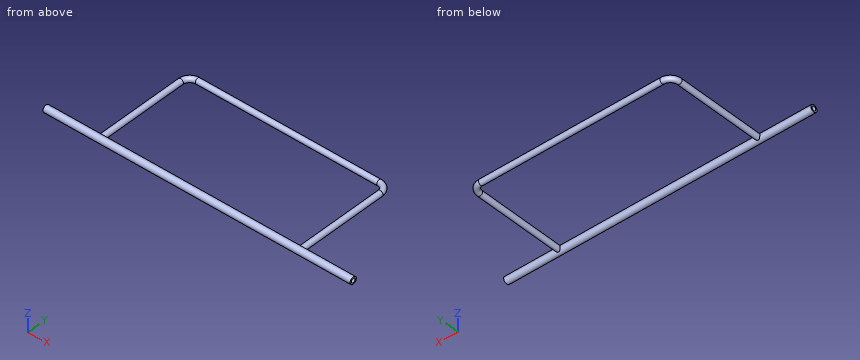
```python
from build123d import *

# Parameters (mm, degrees)
SKETCH1_R           = 5
BOSS_EXTRUDE1_DEPTH = 220
SWEEP1_PROFILE_R    = 4
SKETCH9_R           = 3
CUT_EXTRUDE1_DEPTH  = 220


with BuildPart() as part:
    # Sketch1 → Boss-Extrude1 (new body)
    with BuildSketch(Plane(origin=(0, 0, 0), x_dir=(0, 0, -1), z_dir=(1, 0, 0))):
        Circle(SKETCH1_R)
    boss_extrude1 = extrude(amount=-BOSS_EXTRUDE1_DEPTH)

    # Sweep1: sweep along a path in Sketch2
    with BuildLine(Plane.XY) as sweep1_path:
        Line((-143, 0), (-143, 130))
        ThreePointArc((-143, 130), (-139.192388155, 139.192388155), (-130, 143))
        Line((-130, 143), (0, 143))
    # Sweep1 profile (on start of the path) → Sweep1 (sweep)
    with BuildSketch(Plane(origin=(-143, 0, 0), x_dir=(0, 0, 1), z_dir=(0, 1, 0))):
        Circle(SWEEP1_PROFILE_R)
    sweep1 = sweep(path=sweep1_path.line)

    # Sketch9 → Cut-Extrude1 (cut)
    with BuildSketch(Plane(origin=(0, 0, 0), x_dir=(0, 0, -1), z_dir=(1, 0, 0))):
        Circle(SKETCH9_R)
    cut_extrude1 = extrude(amount=-CUT_EXTRUDE1_DEPTH, mode=Mode.SUBTRACT)

    # Mirror1: Boss-Extrude1, Sweep1, Cut-Extrude1 across plane
    add(boss_extrude1.mirror(Plane(origin=(0, 0, 0), x_dir=(0, 0, 1), z_dir=(1, 0, 0))))
    add(sweep1.mirror(Plane(origin=(0, 0, 0), x_dir=(0, 0, 1), z_dir=(1, 0, 0))))
    add(cut_extrude1.mirror(Plane(origin=(0, 0, 0), x_dir=(0, 0, 1), z_dir=(1, 0, 0))), mode=Mode.SUBTRACT)


solid = part.part
```
Input: part model. Units: mm. Frame: model coordinates. Give positions to 0.01 mm unless a question says otherwise; leave off trailing zeros. Write each loop counter-clockwise with the first axis right and the second up, starting at its lowest first coordinate (ties: lowest second). Pieces come first, ordered by that corner, then holes. Notation, with made-up numbers: (63, -8) - (102, -8) arc R21 cw to (102, 14) - close; hole circle Ø6 at (85.5, 29). An arc over 180 degrees is marked (long way). Write item = value, one per line. Start each with the question number.
1) Cut plane D-D (x = -193). Return loops of the section in (y, z), and give its area (3 significant figures).
2) Cut plane A-A (z = 0). Return loops of the section in (x, y).
3) Cut plane B-B (x = -119.5). Return loops of the section in (y, z).
4) Material intervals for L1, parallel to Y at x = 114, z = 0.5; L2, parallel to Y at x = -137, z = 0; L3, parallel to X at y = 21, z = 0, sorted ascending. Write a range as [from, to].
5) Pin query (flat end, axial travel): pin 1 (1 mm diameter, centred on x = -11.5, z = -2, fed in from -Y); pin 2 (1.5 mm diameter, centred on y = 96.5, z = -3, fed in from -X). Return the tip coordinate at first contact, or that it passes through.
6) Cut plane C-C (y = 74). Return loops of the section in (x, z), and give its area (3 significant figures).
Answers follow:
q1.outline = circle Ø10 at (0, 0); hole circle Ø6 at (0, 0)
q1.area = 50.3 mm^2
q2.outline = (-220, -5) - (220, -5) - (220, -3) - (-220, -3) - close; (-220, 3) - (220, 3) - (220, 5) - (147, 5) - (147, 130) arc R17 ccw to (130, 147) - (-130, 147) arc R17 ccw to (-147, 130) - (-147, 5) - (-220, 5) - close; hole (-139, 5) - (139, 5) - (139, 130) arc R9 ccw to (130, 139) - (-130, 139) arc R9 ccw to (-139, 130) - close
q3.outline = circle Ø10 at (0, 0); circle Ø8 at (143, 0); hole circle Ø6 at (0, 0)
q4.L1 = [-4.97, -2.96], [2.96, 4.97], [139.03, 146.97]
q4.L2 = [-5, -3], [3, 5], [135.66, 145.49]
q4.L3 = [-147, -139], [139, 147]
q5.pin_1 = -4.77
q5.pin_2 = -146.31
q6.outline = circle Ø8 at (-143, 0); circle Ø8 at (143, 0)
q6.area = 101 mm^2
